Verification items for the finished model (mm, model axes). Face numbers are marked on the shaded views. A direction names the side the tool comes from. Coordinates: 2 decimals unless noted, no trailing zeros. Order: outer loops, then holes, each group sorted by start corner. A loop starts at its lowest first (then second) coordinate and runs counter-clockwise, first axis right, second up.
Q1. Draft check along X on the marked faces 4, 5, 6 and 7. Enter one of: pulls with the +X half, pulls with the -X half, needs draft (parallel to the pull), parting line crosses it, or undercut.
Q2. Set-up check for the marked faces 1, 2 and 3: record each of +Z, -Z, +X, -X, +Y, -Y from which the full face is reachable in a straight line by a thin tool's end or side.
Q3. Cross-section at B-B, the plane x = 0. Record the boundary of the cut face in (y, z), and give its area (3 significant figures).
Q4. Depth check by flat-ended pin: P1, Ø2, axis at x = 0, y = 7.5, coming from the +Z side; P2, Ø4, axis at y = -7, z = 5, coming from the +X side; P3, Ø1.1, axis at y = -9, z = 5.5, coming from the -X side. Enter the tip coordinate at first touch or a pass-through.
Q5. Cross-section at D-D, the plane x = -3.5. Record the boundary of the cut face in (y, z).
Q6. Cross-section at C-C, the plane y = 1.75. Record the boundary of the cut face in (x, z), and give its area (3 significant figures).
Q7. Thickness scan on line 1 (Y direction, x = 0, z = 1.5); line 2 (X direction, y = -10.25, z = 6.5); line 3 (Y direction, x = 5.25, z = 4.5). Record the ranges inside material, lowest first.
Q8. Cross-section at A-A, the plane z = 3. Record the boundary of the cut face in (x, y) (3 decimals).
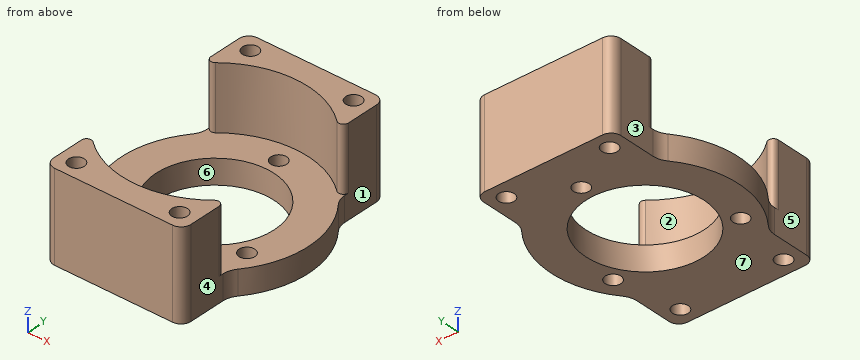
Autodesk Inventor part; units mm, degrees
ref_plane "YZ Plane" through (0, 0, 0) normal (1, 0, 0) x (0, 1, 0)
ref_plane "XZ Plane" through (0, 0, 0) normal (0, 1, 0) x (-1, 0, 0)
ref_plane "XY Plane" through (0, 0, 0) normal (0, 0, 1) x (1, 0, 0)
sketch "スケッチ1" plane through (0, 0, 0) normal (0, 0, 1) x (1, 0, 0)
  circle A0 centre (0, 0) radius 2.5
  circle A1 centre (0, 0) radius 6
  circle A2 centre (0, 0) radius 9.5
  circle A3 centre (0, 7.5) radius 0.8
  circle A4 centre (0, 0) radius 7.5 construction
  line L0 (0, -20.3) -> (0, 20.3)
  circle A5 centre (-6.495191, -3.75) radius 0.8
  circle A6 centre (6.495191, -3.75) radius 0.8
  circle A7 centre (0, 0) radius 14.5 construction
  line L1 (-7, 6.422616) -> (-7, 10.922616)
  line L2 (-6, 11.922616) -> (6, 11.922616)
  line L3 (7, 10.922616) -> (7, 6.422616)
  arc A8 (-6, 11.922616) -> (-7, 10.922616) centre (-6, 10.922616) ccw
  arc A9 (7, 10.922616) -> (6, 11.922616) centre (6, 10.922616) ccw
  circle A10 centre (5.25, 10.231691) radius 2 construction
  circle A11 centre (5.25, 10.231691) radius 0.8
  circle A12 centre (-5.25, 10.231691) radius 2 construction
  circle A13 centre (-5.25, 10.231691) radius 0.8
  line L4 (-5.25, 10.231691) -> (-5.25, 7.917544) construction
  line L5 (5.25, 10.231691) -> (5.25, 7.917544) construction
  circle A14 centre (5.25, -10.231691) radius 0.8
  line L6 (7, -6.422616) -> (7, -10.922616)
  arc A15 (6, -11.922616) -> (7, -10.922616) centre (6, -10.922616) ccw
  line L7 (6, -11.922616) -> (-6, -11.922616)
  circle A16 centre (-5.25, -10.231691) radius 2 construction
  line L8 (-7, -10.922616) -> (-7, -6.422616)
  arc A17 (-7, -10.922616) -> (-6, -11.922616) centre (-6, -10.922616) ccw
  circle A18 centre (-5.25, -10.231691) radius 0.8
  circle A19 centre (5.25, -10.231691) radius 2 construction
  dimension "d4" = 15
  dimension "d0" = 5
  dimension "d1" = 12
  dimension "d2" = 19
  dimension "d3" = 1.6
  dimension "d7" = 360
  dimension "d13" = 29
  dimension "d14" = 1
  dimension "d15" = 12
  dimension "d16" = 4.5
  dimension "d17" = 4
  dimension "d18" = 1.6
  dimension "d19" = 10.5
  dimension "d22" = 360
extrude "押し出し1" add sketch "スケッチ1" along normal blind 1.25 contours L0 A3 A2 A1 | A1 L0 A2 A3
extrude "押し出し2" add sketch "スケッチ1" along normal blind 2.5 contours L0 A3 A2 A1 | A1 L0 A2 A3
extrude "押し出し3" add sketch "スケッチ1" along normal blind 9 contours L0 L7 A17 L8 A2 | A2 L6 A15 L7 L0 | L0 L2 A9 L3 A2 | A2 L1 A8 L2 L0
fillet "フィレット1" radius 2 4 edges at (-7, 6.4226, 1.25) (-7, -6.4226, 1.25) (7, 6.4226, 1.25) (7, -6.4226, 1.25)
fillet "フィレット2" radius 0.5 4 edges at (7, 6.4226, 5.75) (7, -6.4226, 5.75) (-7, -6.4226, 5.75) (-7, 6.4226, 5.75)
properties part number "MotorMount_sub"
Check values:
1. face 4: pulls with the +X half
1. face 5: pulls with the -X half
1. face 6: undercut
1. face 7: needs draft
2. face 1: +Z, -Z, +X, +Y
2. face 2: +Z
2. face 3: +Z, -Z, -X, +Y
3. outline: (-11.92, 0) - (-6, 0) - (-6, 2.5) - (-9.5, 2.5) - (-9.5, 9) - (-11.92, 9) - close; (6, 0) - (6.7, 0) - (6.7, 2.5) - (6, 2.5) - close; (8.3, 0) - (11.92, 0) - (11.92, 9) - (9.5, 9) - (9.5, 2.5) - (8.3, 2.5) - close
3. area: 57.1 mm2
4. P1: stops at z = 2.5
4. P2: stops at x = 7
4. P3: stops at x = -7
5. outline: (-11.92, 0) - (-4.87, 0) - (-4.87, 2.5) - (-8.83, 2.5) - (-8.83, 9) - (-11.92, 9) - close; (4.87, 0) - (11.92, 0) - (11.92, 9) - (8.83, 9) - (8.83, 2.5) - (4.87, 2.5) - close
6. outline: (-9.34, 0) - (-5.74, 0) - (-5.74, 2.5) - (-9.34, 2.5) - close; (5.74, 0) - (9.34, 0) - (9.34, 2.5) - (5.74, 2.5) - close
6. area: 18.0 mm2
7. line 1: y = -11.92 to -6, 6 to 6.7, 8.3 to 11.92
7. line 2: x = -7 to -6.05, -4.45 to 4.45, 6.05 to 7
7. line 3: y = -11.92 to -11.03, -9.43 to -7.92, 7.92 to 9.43, 11.03 to 11.92
8. outline: (-7, -10.923) arc R1 ccw to (-6, -11.923) - (6, -11.923) arc R1 ccw to (7, -10.923) - (7, -7.599) arc R0.5 ccw to (6.175, -7.219) arc R9.5 cw to (-6.175, -7.219) arc R0.5 ccw to (-7, -7.599) - close; (-7, 7.599) arc R0.5 ccw to (-6.175, 7.219) arc R9.5 cw to (6.175, 7.219) arc R0.5 ccw to (7, 7.599) - (7, 10.923) arc R1 ccw to (6, 11.923) - (-6, 11.923) arc R1 ccw to (-7, 10.923) - close; hole circle Ø1.6 at (-5.25, -10.232); hole circle Ø1.6 at (-5.25, 10.232); hole circle Ø1.6 at (5.25, -10.232); hole circle Ø1.6 at (5.25, 10.232)
